CAD build for the part. Positions are in the model's coordinates, mm. A direction names the side the tool comes from. Give positions to 0.01 mm unless a question says otherwise; leave off trailing zeros. Write each loop counter-clockwise with the first axis right and the second up, starting at its lowest first coordinate (ties: lowest second). Pieces come first, ordered by that corner, then holes. Notation, with made-up numbers: (0, 6.5) - (8, 6.5) arc R23 cw to (8, 17.5) - close; hole circle Ø7 at (66.5, 65.25). An arc over 180 degrees is marked (long way). Put each result on its own line as item: value. Start each with the question number.
1. Cut at B-B on x = 28. List the corners of the cut face in (y, z), and give its area (3 significant figures).
2. Drop flat-ended pins along their axis: pin 1 (3 mm diameter, centred on y = -21, z = 27, fed in from -X); pin 2 (8 mm diameter, centred on x = -14.5, z = 11.5, fed in from -Y); pin 3 (3 mm diameter, centred on y = 2, z = 13.5, fed in from -X). Give the stop position or say it passes through.
3. Wall check: line 1 (X direction, y = -1.5, z = 6.5); line 2 (Y direction, x = -39.5, z = 7); line 3 (Y direction, x = -36.5, z = 32). Give the ranges that are in metal, low to high.
4. Cut at A-A on z = 8.5. Give the number of separate pieces and of enclosed holes in the cut face, and give its area (3 significant figures).
5. Tool access for faces 1 (the flat face through (5.3, -22.88, 7.78)), 2 (the flat face through (-12, 5.701, 20)): list every direction of +Z, -Z, +X, -X, +Y, -Y with a clear straight run to the whole face (end or side of a thin tool).
6. Mould opens along Y. For faces 3 (the cylindrical face through (18.455, 6.789, 7.776)), 4 (the flat face through (6.12, 22.72, 7.78)), 5 (the flat face through (-7, 0, 0)) say: +Y half, -Y half, draft (parallel to the pull), parting line (faces both ways), or undercut.
from build123d import *

# Parameters (mm, degrees)
F0_R     = 10.045225
F1_DEPTH = 15.7734
F2_DEPTH = 40.2336
F3_R     = 3.302


with BuildPart() as f1:
    # F0 (on Top) → F1 (new body)
    with BuildSketch(Plane.XY):
        with BuildLine():
            ThreePointArc((-19.276231, 27.17319), (-4.995638, 16.791712), (0.458613, 0))
            ThreePointArc((0.458613, 0), (-5.031754, -16.841329), (-19.39303, -27.210911))
            Line((-19.39303, -27.210911), (30.698986, -18.424801))
            ThreePointArc((30.698986, -18.424801), (44.908516, -0.061007), (30.816896, 18.393421))
            Line((30.816896, 18.393421), (-19.276231, 27.17319))
        make_face()
        with Locations((25.858613, 0)):
            Circle(F0_R, mode=Mode.SUBTRACT)
    extrude(amount=F1_DEPTH)

    # F0 (on Top) → F2 (join)
    with BuildSketch(Plane.XY):
        with BuildLine():
            ThreePointArc((-19.39303, -27.210911), (-5.031754, -16.841329), (0.458613, 0))
            ThreePointArc((0.458613, 0), (-4.995638, 16.791712), (-19.276231, 27.17319))
            ThreePointArc((-19.276231, 27.17319), (-56.691321, 0.061369), (-19.39303, -27.210911))
        make_face()
        with BuildLine():
            ThreePointArc((-14.385945, -3.95065), (-42.37357, -0.930265), (-15.015728, 5.70135))
            Line((-15.015728, 5.70135), (-9.030028, 5.70135))
            Line((-9.030028, 5.70135), (-9.030028, -3.95065))
            Line((-9.030028, -3.95065), (-14.385945, -3.95065))
        make_face(mode=Mode.SUBTRACT)
    extrude(amount=F2_DEPTH)

    # F3
    f3_edges = [f1.edges().sort_by_distance(p)[0] for p in [
        (-36.839744, 27.210911, 40.2336),
    ]]
    fillet(f3_edges, radius=F3_R)


solid = f1.part
Report:
1. outline: (-18.9, 0) - (-9.81, 0) - (-9.81, 15.77) - (-18.9, 15.77) - close; (9.81, 0) - (18.89, 0) - (18.89, 15.77) - (9.81, 15.77) - close
1. area: 286 mm²
2. pin 1: stops at x = -49
2. pin 2: stops at y = -27.05
2. pin 3: stops at x = -56.69
3. line 1: x = -56.65 to -42.32, -9.03 to 15.93, 35.79 to 44.85
3. line 2: y = -26.21 to -8.63, 8.63 to 26.21
3. line 3: y = -27.32 to -11.57, 11.57 to 27.32
4. separate pieces: 1
4. enclosed holes: 2
4. area: 3,440 mm²
5. face 1: +Z, -Z, +X, -Y
5. face 2: +Z, -Z
6. face 3: undercut
6. face 4: +Y half
6. face 5: draft
